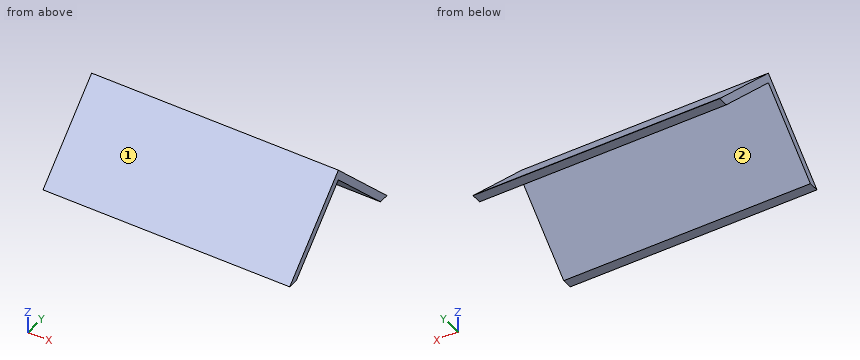
from build123d import *

# Parameters (mm, degrees)
F1_DEPTH = 60
F2_DEPTH = 8.4


with BuildPart() as f1:
    # F0 (on Right) → F1 (new body)
    with BuildSketch(Plane.YZ):
        Polygon((-124.5425649285, 38.5748143829), (-106.5425649285, 56.5748143829), (-88.5425649285, 38.5748143829), (-85.7141378038, 38.5748143829), (-87.1283513662, 39.9890279453), (-106.5425649285, 59.4032415077), (-125.9567784909, 39.9890279453), (-127.3709920533, 38.5748143829), align=None)
    extrude(amount=F1_DEPTH)

    # F2 (add): a face of the model
    f2_faces = [f1.faces().sort_by_distance(p)[0] for p in [
        (0, -125.9567784909, 39.0405521721),
    ]]
    extrude(f2_faces, amount=F2_DEPTH)


solid = f1.part
CAD build for the part. Positions are in the model's coordinates, mm. Face numbers are marked on the shaded views. Round coordinates to 2 decimals unless told otherwise and drop trailing zeros. Write each loop counter-clockwise with the first axis right and the second up, starting at its lowest first coordinate (ties: lowest second). Pieces come first, ordered by that corner, then holes. Notation, with made-up numbers: M 62.5,26 L 68.5,26 A19 cw 68.5,62 Z; hole C 2.5,74.25 d8. An arc over 180 degrees is marked long. Use a Markdown table: item, result. Add a question column.
1. Flat gauge pins, fed straight in: P1, Ø12, axis at x = 7.5, y = -114.5, coming from the +Z side; P2, Ø2, axis at x = 47, y = -109, coming from the +Z side; P3, Ø1.5, axis at x = 51, z = 56.5, coming from the -Y side. Where does each tip first touch, or does it go through?
2. Slice it at C-C on y = -122.5. Give the cut face in (x, z).
3. Slice it at B-B on x = 35.5. Give the cut face in (y, z), then the cut area to 3 significant figures.
4. Drill centre lines: probe 1 along Y at (x, z) = (46.5, 49); probe 2 along Y at (x, z) = (-3.5, 53.5); probe 3 along Z at (x, y) = (37.5, -123). Where is each one in solid material? Low to high.
5. Slice it at A-A on z = 44.75. Give the cut face in (x, y), then the cut area to 3 significant figures.
6. Pull direction Y, two halves, no side cores. Call the marked faces 1 and 2: released by +Y, released by -Y, zero draft, split by the parting line, or undercut.
Reply:
| question | item | result |
|---|---|---|
| 1 | P1 | stops at z = 57.45 |
| 1 | P2 | stops at z = 57.95 |
| 1 | P3 | stops at y = -110.2 |
| 2 | outline | M -8.4,40.62 L 60,40.62 L 60,43.45 L -8.4,43.45 Z |
| 3 | outline | M -127.37,38.57 L -124.54,38.57 L -106.54,56.57 L -88.54,38.57 L -85.71,38.57 L -106.54,59.4 Z |
| 3 | area | 110 mm^2 |
| 4 | probe 1 | y = -116.95 to -114.12, -98.97 to -96.14 |
| 4 | probe 2 | y = -112.45 to -109.62, -103.47 to -100.64 |
| 4 | probe 3 | z = 40.12 to 42.95 |
| 5 | outline | M -8.4,-121.2 L 60,-121.2 L 60,-118.37 L -8.4,-118.37 Z; M -8.4,-94.72 L 60,-94.72 L 60,-91.89 L -8.4,-91.89 Z |
| 5 | area | 387 mm^2 |
| 6 | face 1 | released by -Y |
| 6 | face 2 | undercut |
